Geometry: final body of the model. Coordinates: model frame, mm. A direction names the side the tool comes from. Coordinates: 2 decimals unless noted, no trailing zeros. Write each loop counter-clockwise with the first axis right and the second up, starting at its lowest first coordinate (ties: lowest second). Pieces come first, ordered by that corner, then holes. Notation, with made-up numbers: (32.5, 85.5) -> (75.5, 85.5) arc R16 ccw to (75.5, 94.5) -> close; hole circle Ø9 at (9, 66.5). An arc over 180 degrees is marked (long way). Answer as a JSON object with one key per item and string values. Group by question number.
```python
from build123d import *

# Parameters (mm, degrees)
BOSS_EXTRUDE1_DEPTH = 6
BOSS_EXTRUDE2_START = 1
SKETCH1_3_R         = 16
BOSS_EXTRUDE2_DEPTH = 4
CUT_EXTRUDE2_START  = 5
CUT_EXTRUDE2_DEPTH  = 1
SKETCH1_5_R         = 16
SKETCH1_5_R_2       = 8
BOSS_EXTRUDE3_DEPTH = 6.25
SKETCH2_R           = 18.5
BOSS_EXTRUDE4_DEPTH = 20.75
CUT_EXTRUDE3_START  = 6.25
SKETCH1_6_R         = 8
CUT_EXTRUDE3_DEPTH  = 13
SKETCH3_R           = 5
CUT_EXTRUDE4_DEPTH  = 11


with BuildPart() as part:
    # Sketch1 → Boss-Extrude1 (new body)
    with BuildSketch(Plane(origin=(0, 0, 0), x_dir=(1, 0, 0), z_dir=(0, 1, 0))):
        with BuildLine():
            ThreePointArc((17.805731394, 12.921142733), (19.115621979, 10.890041155), (20.194814379, 8.727512373))
            Line((20.194814379, 8.727512373), (25.139742278, 11.067703815))
            Line((25.139742278, 11.067703815), (24.811761788, 11.742187913))
            ThreePointArc((24.811761788, 11.742187913), (24.686117973, 12.004085947), (24.557709816, 12.264639767))
            ThreePointArc((24.557709816, 12.264639767), (23.484144419, 12.175944584), (22.425086919, 11.978950399))
            ThreePointArc((22.425086919, 11.978950399), (22.239976661, 12.319221327), (22.049703631, 12.656632481))
            ThreePointArc((22.049703631, 12.656632481), (22.778448625, 13.44994215), (23.423080118, 14.312994718))
            ThreePointArc((23.423080118, 14.312994718), (23.270310046, 14.560053928), (23.114934172, 14.805482708))
            ThreePointArc((23.114934172, 14.805482708), (22.056878458, 14.603176993), (21.02475993, 14.294727906))
            ThreePointArc((21.02475993, 14.294727906), (20.804529775, 14.613395117), (20.579470072, 14.928669986))
            ThreePointArc((20.579470072, 14.928669986), (21.21976293, 15.794946243), (21.769005591, 16.721629574))
            ThreePointArc((21.769005591, 16.721629574), (21.590840207, 16.95105068), (21.410257088, 17.178573614))
            ThreePointArc((21.410257088, 17.178573614), (20.379699251, 16.864949571), (19.386214008, 16.448540434))
            ThreePointArc((19.386214008, 16.448540434), (19.133359253, 16.741993301), (18.876062894, 17.031559695))
            ThreePointArc((18.876062894, 17.031559695), (19.420648841, 17.960987283), (19.868279532, 18.940801685))
            ThreePointArc((19.868279532, 18.940801685), (19.666737521, 19.149985255), (19.462993236, 19.357024417))
            ThreePointArc((19.462993236, 19.357024417), (18.471609908, 18.935635532), (17.528014536, 18.415984427))
            ThreePointArc((17.528014536, 18.415984427), (17.245400125, 18.680898012), (16.95878238, 18.941475027))
            ThreePointArc((16.95878238, 18.941475027), (17.401491042, 19.923523161), (17.742437927, 20.945366944))
            ThreePointArc((17.742437927, 20.945366944), (17.519802841, 21.131942845), (17.295205894, 21.316152399))
            ThreePointArc((17.295205894, 21.316152399), (16.354229843, 20.791773177), (15.471215656, 20.174767957))
            ThreePointArc((15.471215656, 20.174767957), (15.162043723, 20.408140683), (14.849352086, 20.636775878))
            ThreePointArc((14.849352086, 20.636775878), (15.185167395, 21.66031756), (15.41556741, 22.712612827))
            ThreePointArc((15.41556741, 22.712612827), (15.174361794, 22.874467079), (14.931456958, 23.033759856))
            ThreePointArc((14.931456958, 23.033759856), (14.05154982, 22.412331723), (13.23912172, 21.704963305))
            ThreePointArc((13.23912172, 21.704963305), (12.906895308, 21.904150965), (12.571672699, 22.098253812))
            ThreePointArc((12.571672699, 22.098253812), (12.796789734, 23.151691906), (12.914032356, 24.222515731))
            ThreePointArc((12.914032356, 24.222515731), (12.656989165, 24.35781446), (12.398528649, 24.49038561))
            ThreePointArc((12.398528649, 24.49038561), (11.589660123, 23.778949595), (10.857023245, 22.989232746))
            ThreePointArc((10.857023245, 22.989232746), (10.505506611, 23.151978465), (10.151551237, 23.309349701))
            ThreePointArc((10.151551237, 23.309349701), (10.263419333, 24.380748332), (10.266176154, 25.457967852))
            ThreePointArc((10.266176154, 25.457967852), (9.996207791, 25.565178071), (9.725120055, 25.66952551))
            ThreePointArc((9.725120055, 25.66952551), (8.996454945, 24.876142467), (8.351910358, 24.013024994))
            ThreePointArc((8.351910358, 24.013024994), (7.985086326, 24.137484798), (7.616408643, 24.256341344))
            ThreePointArc((7.616408643, 24.256341344), (7.613760289, 25.333561137), (7.502000074, 26.404971026))
            ThreePointArc((7.502000074, 26.404971026), (7.222165388, 26.482877999), (6.941521966, 26.557819428))
            ThreePointArc((6.941521966, 26.557819428), (6.301316338, 25.691478704), (5.752166989, 24.764740074))
            ThreePointArc((5.752166989, 24.764740074), (5.374191823, 24.849503783), (4.994969096, 24.928498947))
            ThreePointArc((4.994969096, 24.928498947), (4.877834298, 25.999334571), (4.652823336, 27.052795327))
            ThreePointArc((4.652823336, 27.052795327), (4.366292966, 27.100516337), (4.079273659, 27.145202641))
            ThreePointArc((4.079273659, 27.145202641), (3.5347813, 26.215720222), (3.087249271, 25.235860753))
            ThreePointArc((3.087249271, 25.235860753), (2.702405579, 25.279967961), (2.316934553, 25.318206696))
            ThreePointArc((2.316934553, 25.318206696), (2.086640496, 26.370525157), (1.750928251, 27.394100647))
            ThreePointArc((1.750928251, 27.394100647), (1.460948699, 27.411094996), (1.170805551, 27.425019861))
            ThreePointArc((1.170805551, 27.425019861), (0.728195776, 26.442927155), (0.387351784, 25.421049046))
            ThreePointArc((0.387351784, 25.421049046), (0, 25.424), (-0.387351784, 25.421049046))
            ThreePointArc((-0.387351784, 25.421049046), (-0.728195776, 26.442927155), (-1.170805551, 27.425019861))
            ThreePointArc((-1.170805551, 27.425019861), (-1.460948699, 27.411094996), (-1.750928251, 27.394100647))
            ThreePointArc((-1.750928251, 27.394100647), (-2.086640496, 26.370525157), (-2.316934553, 25.318206696))
            ThreePointArc((-2.316934553, 25.318206696), (-2.702405579, 25.279967961), (-3.087249271, 25.235860753))
            ThreePointArc((-3.087249271, 25.235860753), (-3.5347813, 26.215720222), (-4.079273659, 27.145202641))
            ThreePointArc((-4.079273659, 27.145202641), (-4.366292966, 27.100516337), (-4.652823336, 27.052795327))
            ThreePointArc((-4.652823336, 27.052795327), (-4.877834298, 25.999334571), (-4.994969096, 24.928498947))
            ThreePointArc((-4.994969096, 24.928498947), (-5.374191823, 24.849503783), (-5.752166989, 24.764740074))
            ThreePointArc((-5.752166989, 24.764740074), (-6.301316338, 25.691478704), (-6.941521966, 26.557819428))
            ThreePointArc((-6.941521966, 26.557819428), (-7.222165388, 26.482877999), (-7.502000074, 26.404971026))
            ThreePointArc((-7.502000074, 26.404971026), (-7.613760289, 25.333561137), (-7.616408643, 24.256341344))
            ThreePointArc((-7.616408643, 24.256341344), (-7.985086326, 24.137484798), (-8.351910358, 24.013024994))
            ThreePointArc((-8.351910358, 24.013024994), (-8.996454945, 24.876142467), (-9.725120055, 25.66952551))
            ThreePointArc((-9.725120055, 25.66952551), (-9.996207791, 25.565178071), (-10.266176154, 25.457967852))
            ThreePointArc((-10.266176154, 25.457967852), (-10.263419333, 24.380748332), (-10.151551237, 23.309349701))
            ThreePointArc((-10.151551237, 23.309349701), (-10.505506611, 23.151978465), (-10.857023245, 22.989232746))
            ThreePointArc((-10.857023245, 22.989232746), (-11.589660123, 23.778949595), (-12.398528649, 24.49038561))
            ThreePointArc((-12.398528649, 24.49038561), (-12.656989165, 24.35781446), (-12.914032356, 24.222515731))
            ThreePointArc((-12.914032356, 24.222515731), (-12.796789734, 23.151691906), (-12.571672699, 22.098253812))
            ThreePointArc((-12.571672699, 22.098253812), (-12.906895308, 21.904150965), (-13.23912172, 21.704963305))
            ThreePointArc((-13.23912172, 21.704963305), (-14.05154982, 22.412331723), (-14.931456958, 23.033759856))
            ThreePointArc((-14.931456958, 23.033759856), (-15.174361794, 22.874467079), (-15.41556741, 22.712612827))
            ThreePointArc((-15.41556741, 22.712612827), (-15.185167395, 21.66031756), (-14.849352086, 20.636775878))
            ThreePointArc((-14.849352086, 20.636775878), (-15.162043723, 20.408140683), (-15.471215656, 20.174767957))
            ThreePointArc((-15.471215656, 20.174767957), (-16.354229843, 20.791773177), (-17.295205894, 21.316152399))
            ThreePointArc((-17.295205894, 21.316152399), (-17.519802841, 21.131942845), (-17.742437927, 20.945366944))
            ThreePointArc((-17.742437927, 20.945366944), (-17.401491042, 19.923523161), (-16.95878238, 18.941475027))
            ThreePointArc((-16.95878238, 18.941475027), (-17.245400125, 18.680898012), (-17.528014536, 18.415984427))
            ThreePointArc((-17.528014536, 18.415984427), (-18.471609908, 18.935635532), (-19.462993236, 19.357024417))
            ThreePointArc((-19.462993236, 19.357024417), (-19.666737521, 19.149985255), (-19.868279532, 18.940801685))
            ThreePointArc((-19.868279532, 18.940801685), (-19.420648841, 17.960987283), (-18.876062894, 17.031559695))
            ThreePointArc((-18.876062894, 17.031559695), (-19.133359253, 16.741993301), (-19.386214008, 16.448540434))
            ThreePointArc((-19.386214008, 16.448540434), (-20.379699251, 16.864949571), (-21.410257088, 17.178573614))
            ThreePointArc((-21.410257088, 17.178573614), (-21.590840207, 16.95105068), (-21.769005591, 16.721629574))
            Line((-21.769005591, 16.721629574), (-22.232149052, 16.131715907))
            Line((-22.232149052, 16.131715907), (-17.893635567, 12.799133025))
            ThreePointArc((-17.893635567, 12.799133025), (-0.07518895, 21.999871514), (17.805731394, 12.921142733))
        make_face()
    extrude(amount=BOSS_EXTRUDE1_DEPTH)

    # Sketch1<3> → Boss-Extrude2 (add)
    with BuildSketch(Plane(origin=(0, 0, 0), x_dir=(1, 0, 0), z_dir=(0, 1, 0)).offset(BOSS_EXTRUDE2_START)):
        with BuildLine():
            ThreePointArc((17.928788602, 1.599543458), (17.447292969, 4.426281516), (16.523029946, 7.140691941))
            ThreePointArc((16.523029946, 7.140691941), (15.640054347, 8.910033672), (14.568325686, 10.571844055))
            Line((14.568325686, 10.571844055), (15.377677113, 11.159168724))
            Line((15.377677113, 11.159168724), (17.805731394, 12.921142733))
            ThreePointArc((17.805731394, 12.921142733), (-0.07518895, 21.999871514), (-17.893635567, 12.799133025))
            ThreePointArc((-17.893635567, 12.799133025), (-5.782522672, -21.226455935), (21.912963847, 1.954997559))
            Line((21.912963847, 1.954997559), (17.928788602, 1.599543458))
        make_face()
        Circle(SKETCH1_3_R, mode=Mode.SUBTRACT)
        with BuildLine():
            ThreePointArc((14.568325686, 10.571844055), (15.640054347, 8.910033672), (16.523029946, 7.140691941))
            Line((16.523029946, 7.140691941), (20.194814379, 8.727512373))
            ThreePointArc((20.194814379, 8.727512373), (19.115621979, 10.890041155), (17.805731394, 12.921142733))
            Line((17.805731394, 12.921142733), (15.377677113, 11.159168724))
            Line((15.377677113, 11.159168724), (14.568325686, 10.571844055))
        make_face()
    extrude(amount=BOSS_EXTRUDE2_DEPTH)

    # Sketch1<4> → Cut-Extrude2 (cut)
    with BuildSketch(Plane(origin=(0, 0, 0), x_dir=(1, 0, 0), z_dir=(0, 1, 0)).offset(CUT_EXTRUDE2_START)):
        with BuildLine():
            ThreePointArc((14.568325686, 10.571844055), (15.640054347, 8.910033672), (16.523029946, 7.140691941))
            Line((16.523029946, 7.140691941), (20.194814379, 8.727512373))
            ThreePointArc((20.194814379, 8.727512373), (19.115621979, 10.890041155), (17.805731394, 12.921142733))
            Line((17.805731394, 12.921142733), (15.377677113, 11.159168724))
            Line((15.377677113, 11.159168724), (14.568325686, 10.571844055))
        make_face()
    extrude(amount=-CUT_EXTRUDE2_DEPTH, mode=Mode.SUBTRACT)

    # Sketch1<5> → Boss-Extrude3 (add)
    with BuildSketch(Plane(origin=(0, 0, 0), x_dir=(1, 0, 0), z_dir=(0, 1, 0))):
        Circle(SKETCH1_5_R)
        Circle(SKETCH1_5_R_2, mode=Mode.SUBTRACT)
    extrude(amount=BOSS_EXTRUDE3_DEPTH)

    # Sketch2 → Boss-Extrude4 (add)
    with BuildSketch(Plane.XZ.offset(-1)):
        Circle(SKETCH2_R)
    extrude(amount=BOSS_EXTRUDE4_DEPTH)

    # Sketch1<6> → Cut-Extrude3 (cut)
    with BuildSketch(Plane(origin=(0, 0, 0), x_dir=(1, 0, 0), z_dir=(0, 1, 0)).offset(CUT_EXTRUDE3_START)):
        Circle(SKETCH1_6_R)
    extrude(amount=-CUT_EXTRUDE3_DEPTH, mode=Mode.SUBTRACT)

    # Sketch3 → Cut-Extrude4 (cut)
    with BuildSketch(Plane.XZ.offset(19.75)):
        Circle(SKETCH3_R)
    extrude(amount=-CUT_EXTRUDE4_DEPTH, mode=Mode.SUBTRACT)


solid = part.part
```
Item 1: Section C-C on z = 7. Output: boundary loops of the cut face in (x, y), then the cut area to 3 significant figures.
Item 2: Section A-A on y = -3.25. Output: boundary loops of the cut face in (x, z), then the cut area to 3 significant figures.
Item 3: Ray query, L1, parallel to X at y = 2.5, z = 0; L2, parallel to X at y = -2.5, z = 0. Return the intervals inside material, ascending. Write a range as [from, to].
Item 4: Section B-B on z = 0. Output: boundary loops of the cut face in (x, y), then the cut area to 3 significant figures.
Item 5: Set-up query: faces 1 (the flat face through (17, 4, -10)), 2 (the cylindrical face through (22.072, 2.958, -14.607)), 3 (the cylindrical face through (9.01, 2.96, -24.89)). Return all of +Z, -Z, +X, -X, +Y, -Y with unobstructed straight access to the full face (end or side cutting, diameter ignored); none if empty.
Item 6: Section D-D on y = -11. Output: boundary loops of the cut face in (x, z), then the cut area to 3 significant figures.
Item 7: Contact query for flat-ended pins moving along their axis: pin 1 (5 mm diameter, centred on x = -7.5, y = -10.5, fed in from -Z); pin 2 (4.5 mm diameter, centred on x = 17.5, z = -10, fed in from +Y); pin 3 (4 mm diameter, centred on x = 19.5, y = 3, fed in from +Z). Output: stop coordinate, or through.
Item 8: Mould query, pull axis Z, two halves, no side actions, for faces 4 (the cylindrical face through (-11.58, 2.96, -23.77)), 5 (the flat face through (0, -8.75, 0)), 6 (the flat face through (-3.8, 6.25, -7.3)). Classes: +Z half, -Z half, draft (parallel to the pull), parting line (faces both ways), or undercut.
Answer sheet:
{
 "1": {"outline": "(-20.86, 1) -> (-17.12, 1) -> (-17.12, -19.75) -> (17.12, -19.75) -> (17.12, 1) -> (20.86, 1) -> (20.86, 5) -> (14.39, 5) -> (14.39, 6.25) -> (3.87, 6.25) -> (3.87, -6.75) -> (-3.87, -6.75) -> (-3.87, 6.25) -> (-14.39, 6.25) -> (-14.39, 5) -> (-20.86, 5) -> close", "area": "813 mm^2"},
 "2": {"outline": "circle Ø37 at (0, 0); hole circle Ø16 at (0, 0)", "area": "874 mm^2"},
 "3": {"L1": "x = [-22, -8], [8, 22]", "L2": "x = [-18.5, -8], [8, 18.5]"},
 "4": {"outline": "(-22, 1) -> (-18.5, 1) -> (-18.5, -19.75) -> (-5, -19.75) -> (-5, -8.75) -> (5, -8.75) -> (5, -19.75) -> (18.5, -19.75) -> (18.5, 1) -> (22, 1) -> (22, 5) -> (16, 5) -> (16, 6.25) -> (8, 6.25) -> (8, -6.75) -> (-8, -6.75) -> (-8, 6.25) -> (-16, 6.25) -> (-16, 5) -> (-22, 5) -> close", "area": "666 mm^2"},
 "5": {"face 1": "+Y", "face 2": "+Y, -Y", "face 3": "-Z, +Y, -Y"},
 "6": {"outline": "circle Ø37 at (0, 0); hole circle Ø10 at (0, 0)", "area": "997 mm^2"},
 "7": {"pin 1": "stops at z = -17.81", "pin 2": "stops at y = 6", "pin 3": "stops at z = 13.33"},
 "8": {"face 4": "-Z half", "face 5": "undercut", "face 6": "draft"}
}
